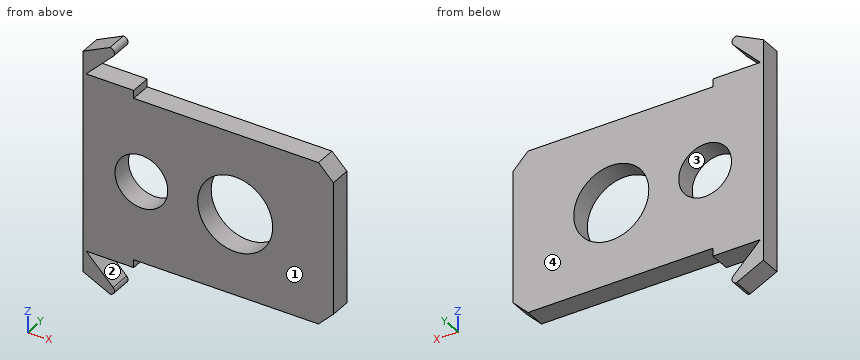
from build123d import *

# Parameters (mm, degrees)
SKETCH3_R           = 1
SKETCH3_R_2         = 1.421368712
BOSS_EXTRUDE1_DEPTH = 0.8


with BuildPart() as part:
    # Sketch3 → Boss-Extrude1 (new body)
    with BuildSketch(Plane(origin=(0, 0, 0), x_dir=(1, 0, 0), z_dir=(0, 1, 0))):
        with BuildLine():
            Line((40.65499317, -3.365685425), (42.45499317, -3.365685425))
            Line((42.45499317, -3.365685425), (42.45499317, -3.065685425))
            Line((42.45499317, -3.065685425), (49.45499317, -3.065685425))
            Line((49.45499317, -3.065685425), (50.020678594, -2.5))
            Line((50.020678594, -2.5), (50.020678594, 2.5))
            Line((50.020678594, 2.5), (49.45499317, 3.065685425))
            Line((49.45499317, 3.065685425), (42.45499317, 3.065685425))
            Line((42.45499317, 3.065685425), (42.45499317, 3.365685425))
            Line((42.45499317, 3.365685425), (40.65499317, 3.365685425))
            Line((40.65499317, 3.365685425), (41.67730974, 4.388001996))
            ThreePointArc((41.67730974, 4.388001996), (41.714807471, 4.576515818), (41.55499317, 4.68330032))
            Line((41.55499317, 4.68330032), (40.539309151, 4.188808518))
            Line((40.539309151, 4.188808518), (40.539309151, -4.188808518))
            Line((40.539309151, -4.188808518), (41.55499317, -4.68330032))
            ThreePointArc((41.55499317, -4.68330032), (41.714807471, -4.576515818), (41.67730974, -4.388001996))
            Line((41.67730974, -4.388001996), (40.65499317, -3.365685425))
        make_face()
        with Locations(Location((42.746488922, 0, 0), (0, 0, 270))):
            Circle(SKETCH3_R, mode=Mode.SUBTRACT)
        with Locations(Location((46.301021107, 0, 0), (0, 0, 270))):
            Circle(SKETCH3_R_2, mode=Mode.SUBTRACT)
    extrude(amount=BOSS_EXTRUDE1_DEPTH)


solid = part.part
Could you check a few things on this model? Use its own coordinates, in mm. Face numbers are marked on the shaded views. A direction names the side the tool comes from. Coordinates: 2 decimals unless noted, no trailing zeros. Order: outer loops, then holes, each group sorted by start corner. A loop starts at its lowest first (then second) coordinate and runs counter-clockwise, first axis right, second up. Notation, with made-up numbers: (-38, 1) -> (19, 1) arc R24 cw to (19, 22) -> close; hole circle Ø9 at (64, -13). An arc over 180 degrees is marked (long way). One line per item, written item: value. Start each with the question number.
1) Which directions (+Z, -Z, +X, -X, +Y, -Y) give clear straight access to the entire face, cutting with the end or side of a thin tool? Please do the marked faces 1 and 2.
2) Imagine slicing it at A-A on z = 0. List the corners of the cut face in (x, y) for me.
3) Imagine slicing it at D-D on x = 48. List the corners of the cut face in (y, z) for me, plus the area to 3 significant figures.
4) We'd pull the mould along Z, two halves only. Please class the marked faces 3 and 4: +Z half, -Z half, draft (parallel to the pull), parting line (faces both ways), or undercut.
5) Imagine slicing it at C-C on y = 0.25. List the corners of the cut face in (x, z) for me (3 decimals).
6) If I drill on L1, parallel to X at y = 0.6, z = 0; L2, parallel to Z at x = 42.75, y = 0.45; L3, parallel to X at y = 0.1, z = -0.5, over which ranges is the centre line in solid material (lowest first)? Write a range as [from, to].
7) Imagine slicing it at B-B on x = 46.5. List the corners of the cut face in (y, z) for me.
Answer list:
1. face 1: +Z, -Z, +X, -X, -Y
1. face 2: +X, +Y, -Y
2. outline: (40.54, 0) -> (41.75, 0) -> (41.75, 0.8) -> (40.54, 0.8) -> close; (43.75, 0) -> (44.88, 0) -> (44.88, 0.8) -> (43.75, 0.8) -> close; (47.72, 0) -> (50.02, 0) -> (50.02, 0.8) -> (47.72, 0.8) -> close
3. outline: (0, -3.07) -> (0.8, -3.07) -> (0.8, 3.07) -> (0, 3.07) -> close
3. area: 4.91 mm2
4. face 3: undercut
4. face 4: draft
5. outline: (40.539, -4.189) -> (41.555, -4.683) arc R0.173 ccw to (41.677, -4.388) -> (40.655, -3.366) -> (42.455, -3.366) -> (42.455, -3.066) -> (49.455, -3.066) -> (50.021, -2.5) -> (50.021, 2.5) -> (49.455, 3.066) -> (42.455, 3.066) -> (42.455, 3.366) -> (40.655, 3.366) -> (41.677, 4.388) arc R0.173 ccw to (41.555, 4.683) -> (40.539, 4.189) -> close; hole circle Ø2 at (42.746, 0); hole circle Ø2.843 at (46.301, 0)
6. L1: x = [40.54, 41.75], [43.75, 44.88], [47.72, 50.02]
6. L2: z = [-3.07, -1], [1, 3.07]
6. L3: x = [40.54, 41.88], [43.61, 44.97], [47.63, 50.02]
7. outline: (0, -3.07) -> (0.8, -3.07) -> (0.8, -1.41) -> (0, -1.41) -> close; (0, 1.41) -> (0.8, 1.41) -> (0.8, 3.07) -> (0, 3.07) -> close
